The model under review builds one solid part; all positions refer to its coordinate system, in mm. A direction names the side the tool comes from. Give positions to 0.01 mm unless a question says otherwise; leave off trailing zeros. Loops run counter-clockwise (first coordinate to the right, second up) from the corner with the lowest first, then second, coordinate; pieces in that order, holes last. Notation, with made-up numbers: M 14,22 L 66,22 A20 ccw 66,58 Z; hole C 74.5,32.5 d1. An arc over 180 degrees is marked long. Return JSON: item names as keys, results as strings.
```python
from build123d import *

# Parameters (mm, degrees)
REVOLVE1_ANGLE = 10


with BuildPart() as part:
    # Sketch2 → Revolve1 (revolve)
    with BuildSketch(Plane.XY):
        with BuildLine():
            ThreePointArc((55, -18.250226729), (44.849284803, -17.402430783), (35, -20))
            Line((35, -20), (35, 20))
            ThreePointArc((35, 20), (52.721414573, 2.677196604), (76.584109665, -4.008596909))
            ThreePointArc((76.584109665, -4.008596909), (76.270130447, -47.769342724), (64.795242944, -90))
            Line((64.795242944, -90), (59.795242944, -90))
            ThreePointArc((59.795242944, -90), (60.100118063, -53.944497774), (55, -18.250226729))
        make_face()
        Polygon((16, -9.25), (35, -9.25), (35, 9.25), (16, 9.25), (16, 0), align=None)
    revolve(axis=Axis((0, 0, 0), (0, -1, 0)), revolution_arc=REVOLVE1_ANGLE)


solid = part.part
```
1) Tool access review of faces 1 (the face through (34.87, -14.55, 3.01)), 2 (the face through (62, -90, 6)), 3 (the face through (34.87, 14.7, 3.01)): name each direction out of +Z, -Z, +X, -X, +Y, -Y from which nothing blocks a thin tool from reaching the whole face with its end or side.
From the geometry:
{"face 1": "-Z, -X, -Y", "face 2": "+Z, -Z, +X, -X, -Y", "face 3": "-Z, -X, +Y"}
2) Insertion check: pin 1 (6 mm diameter, centred on x = 66.5, z = 11, fed in from +Y); pin 2 (8 mm diameter, centred on x = 56.5, z = 5, fed in from +Y); pin 3 (5 mm diameter, centred on x = 43.5, z = 1.5, fed in from +Y). Each pin has a flat end and moves straight along its axis. Give the tip position at first contact, or say it passes through.
From the geometry:
{"pin 1": "y = -2.22", "pin 2": "y = 2.68", "pin 3": "y = 12.02"}
3) Consider section B-B on x = 24. Write out the cut boundary in (y, z), then the cut area to 3 significant figures.
From the geometry:
{"outline": "M -9.25,0 L 9.25,0 L 9.25,4.23 L -9.25,4.23 Z", "area": "78.3 mm²"}
4) Wall thickness on L1, parallel to Y at x = 21.5, z = 1.75; L2, parallel to Z at x = 67.5, y = -51; L3, parallel to X at y = -40, z = 4.75: over which ranges is each line inside the solid? List them lowest first. Write a range as from..to.
From the geometry:
{"L1": "-9.25..9.25", "L2": "0..11.9", "L3": "58.57..77.01"}
5) Consider section A-A on y = 4. Write out the cut boundary in (x, z).
From the geometry:
{"outline": "M 15.76,2.78 A16 cw 16,0 L 50.56,0 A50.56 ccw 49.79,8.78 Z"}
